Autodesk Inventor part; units mm, degrees
ref_plane "Work Plane1" through (-69.5213, -7.1863, -89) normal (0, -1, 0) x (1, 0, 0)
ref_plane "YZ Plane" through (0, 0, 0) normal (1, 0, 0) x (0, 1, 0)
ref_plane "XZ Plane" through (0, 0, 0) normal (0, 1, 0) x (-1, 0, 0)
sketch "Sketch1" plane through (0, 0, 0) normal (0, 0, 1) x (1, 0, 0)
  line L0 (-60.5213, -2.6863) -> (-60.5213, -7.1863)
  line L1 (-69.5213, -2.6863) -> (-60.5213, -2.6863)
  line L2 (-69.5213, -7.1863) -> (-69.5213, -2.6863)
  line L3 (-60.5213, -7.1863) -> (-69.5213, -7.1863)
  line L4 (-60.5213, -7.1863) -> (-58.5213, -7.1863)
  line L5 (-58.5213, -2.6863) -> (-60.5213, -2.6863)
  line L6 (-58.5213, -10.6863) -> (-54.5213, -10.6863)
  line L7 (-54.5213, -10.6863) -> (-54.5213, -7.1863)
  line L8 (-58.5213, -7.1863) -> (-54.5213, -7.1863)
  line L9 (-58.5213, -10.6863) -> (-58.5213, -7.1863)
  line L10 (-58.5213, -2.6863) -> (-58.5213, -7.1863)
  line L11 (-58.5213, -7.1863) -> (-54.5213, -7.1863)
  line L12 (-54.5213, -7.1863) -> (-54.5213, -10.6863)
  line L13 (-54.5213, -10.6863) -> (-40.5213, -10.6863)
  line L14 (-40.5213, -10.6863) -> (-54.5213, -1.6863)
  line L15 (-54.5213, -1.6863) -> (-54.5213, -2.6863)
  line L16 (-54.5213, -2.6863) -> (-58.5213, -2.6863)
  line L17 (-58.5213, -0.9637) -> (-44.5213, -0.9637)
  line L18 (-44.5213, -0.9637) -> (-44.5213, -10.9637)
  line L19 (-44.5213, -10.9637) -> (-58.5213, -10.9637)
  line L20 (-58.5213, -10.9637) -> (-58.5213, -0.9637)
  line L21 (-69.5213, -2.6863) -> (-58.5213, -2.6863)
  line L22 (-58.5213, -2.6863) -> (-58.5213, -7.1863)
  line L23 (-58.5213, -7.1863) -> (-69.5213, -7.1863)
  line L24 (-69.5213, -7.1863) -> (-69.5213, -2.6863)
  circle A0 centre (-213.5213, 2.3137) radius 25
  line L25 (-213.5213, -22.6863) -> (-44.5213, -10.9637)
  line L26 (-213.5213, -22.6863) -> (-213.5213, 2.3137)
  line L27 (-44.5213, -10.9637) -> (-40.5213, -10.6863)
  line L28 (-44.5213, -10.9637) -> (-45.5667, -0.9637)
  line L29 (-58.5213, -2.6863) -> (-54.5213, -2.6863)
  line L30 (-54.5213, -2.6863) -> (-54.5213, -0.9637)
  line L31 (-54.5213, -0.9637) -> (-58.5213, -0.9637)
  line L32 (-58.5213, -0.9637) -> (-58.5213, -2.6863)
  line L33 (-54.5213, -2.6863) -> (-50.5667, -0.9637)
  line L34 (-54.5213, -10.6863) -> (-54.5213, -10.9637)
  point P0 (0, 0)
  point P1 (-53.594, -2.2824)
  point P2 (-44.5503, -10.6863)
  dimension "d0" = 14
  dimension "d1" = 10
  dimension "d3" = 88
  dimension "d15" = 5
  dimension "d16" = 23.537
extrude "Extrusion1" add sketch "Sketch1" along normal mid plane 178 contours L16 L33 L14 L28 L13 L7 L8 L10 | L33 L17 L28 L14 | L13 L28 L19 L34
sketch "Sketch2" plane through (-58.5213, -2.6863, 89) normal (0, 1, 0) x (1, 0, 0)
  circle A0 centre (-4, 67.5) radius 1.2295
  circle A1 centre (-4, 153.5) radius 1.2295
  circle A2 centre (-4, 110.5) radius 1.2295
  circle A3 centre (-4, 24.5) radius 1.2295
  line L0 (-2, 161) -> (-11, 161)
  line L1 (-11, 161) -> (-11, 146)
  line L2 (-11, 146) -> (-2, 146)
  arc A4 (0, 144) -> (-2, 146) centre (-2, 144) ccw
  line L3 (0, 144) -> (0, 120)
  arc A5 (-2, 118) -> (0, 120) centre (-2, 120) ccw
  line L4 (-2, 118) -> (-11, 118)
  line L5 (-11, 118) -> (-11, 103)
  line L6 (-11, 103) -> (-2, 103)
  arc A6 (0, 101) -> (-2, 103) centre (-2, 101) ccw
  line L7 (0, 101) -> (0, 77)
  arc A7 (-2, 75) -> (0, 77) centre (-2, 77) ccw
  line L8 (-2, 75) -> (-11, 75)
  line L9 (-11, 75) -> (-11, 60)
  line L10 (-11, 60) -> (-2, 60)
  arc A8 (0, 58) -> (-2, 60) centre (-2, 58) ccw
  line L11 (0, 58) -> (0, 34)
  arc A9 (-2, 32) -> (0, 34) centre (-2, 34) ccw
  line L12 (-2, 32) -> (-11, 32)
  line L13 (-11, 32) -> (-11, 17)
  line L14 (-11, 17) -> (-2, 17)
  arc A10 (0, 15) -> (-2, 17) centre (-2, 15) ccw
  line L15 (0, 15) -> (0, 0)
  line L16 (4, 0) -> (0, 0)
  line L17 (4, 178) -> (4, 0)
  line L18 (4, 178) -> (0, 178)
  line L19 (0, 178) -> (0, 163)
  arc A11 (-2, 161) -> (0, 163) centre (-2, 163) ccw
  line L20 (0, 178) -> (0, 0)
  point P0 (58.5213, 89)
ref_plane "Work Plane1" through (-69.5213, -7.1863, -89) normal (0, -1, 0) x (1, 0, 0)
extrude "Extrusion2" add sketch "Sketch2" against normal up to surface (4.5 mm away) contours A0 | A1 | A2 | A3 | A11 L20 A4 L2 L1 L0 | L20 A6 L6 L5 L4 A5 | L20 A8 L10 L9 L8 A7 | A10 L14 L13 L12 A9 L20
sketch "Sketch3" plane through (-69.5213, -7.1863, -57) normal (0, -1, 0) x (1, 0, 0)
  circle A0 centre (7, 78.5) radius 1.2295
  circle A1 centre (7, -7.5) radius 1.2295
  circle A2 centre (7, 35.5) radius 1.2295
  circle A3 centre (7, 121.5) radius 1.2295
  line L0 (9, -15) -> (0, -15)
  line L1 (0, -15) -> (0, 0)
  line L2 (0, 0) -> (9, 0)
  arc A4 (9, 0) -> (11, 2) centre (9, 2) ccw
  line L3 (11, 2) -> (11, 26)
  arc A5 (11, 26) -> (9, 28) centre (9, 26) ccw
  line L4 (9, 28) -> (0, 28)
  line L5 (0, 28) -> (0, 43)
  line L6 (0, 43) -> (9, 43)
  arc A6 (9, 43) -> (11, 45) centre (9, 45) ccw
  line L7 (11, 45) -> (11, 69)
  arc A7 (11, 69) -> (9, 71) centre (9, 69) ccw
  line L8 (9, 71) -> (0, 71)
  line L9 (0, 71) -> (0, 86)
  line L10 (0, 86) -> (9, 86)
  arc A8 (9, 86) -> (11, 88) centre (9, 88) ccw
  line L11 (11, 88) -> (11, 112)
  arc A9 (11, 112) -> (9, 114) centre (9, 112) ccw
  line L12 (9, 114) -> (0, 114)
  line L13 (0, 114) -> (0, 129)
  line L14 (0, 129) -> (9, 129)
  arc A10 (9, 129) -> (11, 131) centre (9, 131) ccw
  line L15 (11, 131) -> (11, 146)
  line L16 (15, 146) -> (11, 146)
  line L17 (15, -32) -> (15, 146)
  line L18 (15, -32) -> (11, -32)
  line L19 (11, -32) -> (11, -17)
  arc A11 (11, -17) -> (9, -15) centre (9, -17) ccw
  point P0 (69.5213, 57)
hole "Hole1" at (-62.5213, -7.1863, -64.5) at (-62.5213, -7.1863, -21.5) at (-62.5213, -7.1863, 21.5) at (-62.5213, -7.1863, 64.5) direction (0, 1, 0) diameter 3.9 depth 4.5 counterbore diameter 4.6 counterbore depth 0.75
properties part number "plaski_plog" material "PC/ABS Plastic"
CAD build for the part. Positions are in the model's coordinates, mm. A direction names the side the tool comes from. Round coordinates to 2 decimals unless told otherwise and drop trailing zeros. Write each loop counter-clockwise with the first axis right and the second up, starting at its lowest first coordinate (ties: lowest second). Pieces come first, ordered by that corner, then holes. Notation, with made-up numbers: M 79.5,56 L 132.5,56 A29 ccw 132.5,80 Z; hole C 77.5,45 d11. An arc over 180 degrees is marked long. Use a Markdown table: item, result. Add a question column.
1. Slice it at C-C on y = -4.5. Give the number of separate pieces and of enclosed holes in the cut face, then the cut area to 3 significant figures.
2. Flat gauge pins, fed straight in: P1, Ø2, axis at x = -63, y = -4.5, coming from the +Z side; P2, Ø1.5, axis at x = -56.5, z = -13.5, coming from the -Y side; P3, Ø5, axis at x = -62.52, z = -21.5, coming from the +Y side. Where does each tip first touch, or does it go through?
3. Slice it at A-A on z = 2. Give the cut face in (x, y), then the cut area to 3 significant figures.
4. Pull direction X, two halves, no side cores. Call faces 1 (the face through (-58.521, -5, 81)), 2 (the face through (-48, -0.964, -1)), 3 (the face through (-64.455, -4.535, -21.246)): released by +X, released by -X, zero draft, split by the parting line, or undercut.
5. 3-axis set-ups, long thin cutter, end or side, ignore diameter. For faces 4 (the face through (-57, -7.186, -1)), 5 (the face through (-64, -6.436, 66)), 6 (the face through (-58.521, -5, -82)), 7 (the face through (-50, -6, -89)), 8 (the face through (-65, -5, 14)): which of +Z, -Z, +X, -X, +Y, -Y reach the whole face in a straight line?
6. Slice it at B-B on z = 64.5. Give the cut face in (x, y), then the cut area to 3 significant figures.
7. Slice it at D-D on z = -60. Give the cut face in (x, y).
8. Drill centre lines: probe 1 along Z at (x, y) = (-64.75, -5); probe 2 along X at (y, z) = (-3.85, -21.5); probe 3 along Y at (x, z) = (-57.75, -17.5). Where is each one in solid material? Low to high.
Reply:
| question | item | result |
|---|---|---|
| 1 | separate pieces | 1 |
| 1 | enclosed holes | 4 |
| 1 | area | 2,990 mm^2 |
| 2 | P1 | stops at z = 72 |
| 2 | P2 | stops at y = -7.19 |
| 2 | P3 | stops at y = -2.69 |
| 3 | outline | M -58.52,-7.19 L -54.52,-7.19 L -54.52,-10.96 L -44.52,-10.96 L -45.57,-0.96 L -50.57,-0.96 L -54.52,-2.69 L -58.52,-2.69 Z |
| 3 | area | 109 mm^2 |
| 4 | face 1 | released by -X |
| 4 | face 2 | zero draft |
| 4 | face 3 | undercut |
| 5 | face 4 | +Z, -Z, -X, -Y |
| 5 | face 5 | -Y |
| 5 | face 6 | -Z, -X, +Y, -Y |
| 5 | face 7 | -Z, +X, -X, +Y, -Y |
| 5 | face 8 | -X, +Y, -Y |
| 6 | outline | M -69.52,-7.19 L -64.82,-7.19 L -64.82,-6.44 L -64.47,-6.44 L -64.47,-2.69 L -69.52,-2.69 Z; M -60.57,-6.44 L -60.22,-6.44 L -60.22,-7.19 L -54.52,-7.19 L -54.52,-10.96 L -44.52,-10.96 L -45.57,-0.96 L -50.57,-0.96 L -54.52,-2.69 L -60.57,-2.69 Z |
| 6 | area | 141 mm^2 |
| 7 | outline | M -69.52,-7.19 L -54.52,-7.19 L -54.52,-10.96 L -44.52,-10.96 L -45.57,-0.96 L -50.57,-0.96 L -54.52,-2.69 L -69.52,-2.69 Z |
| 8 | probe 1 | z = -72 to -57, -29 to -14, 14 to 29, 57 to 72 |
| 8 | probe 2 | x = -69.52 to -64.47, -60.57 to -45.26 |
| 8 | probe 3 | y = -7.19 to -2.69 |
